Geometry: see drawing. Coordinates: mm, zero at the bounding-box minimum. Round coordinates to 2 decimals unless told otherwise and drop trailing zeros. Write each loop counter-clockwise with the first axis right and the second up, starting at its lowest first coordinate (ties: lowest second). Pieces come first, ordered by that corner, then holes. Notation, with made-up numbers: (45, 42.5) -> (94, 42.5) arc R8 cw to (94, 49.5) -> close; hole circle Ø1 at (-4, 57.25). An arc over 180 degrees is marked (long way). Write item = value, one per line.
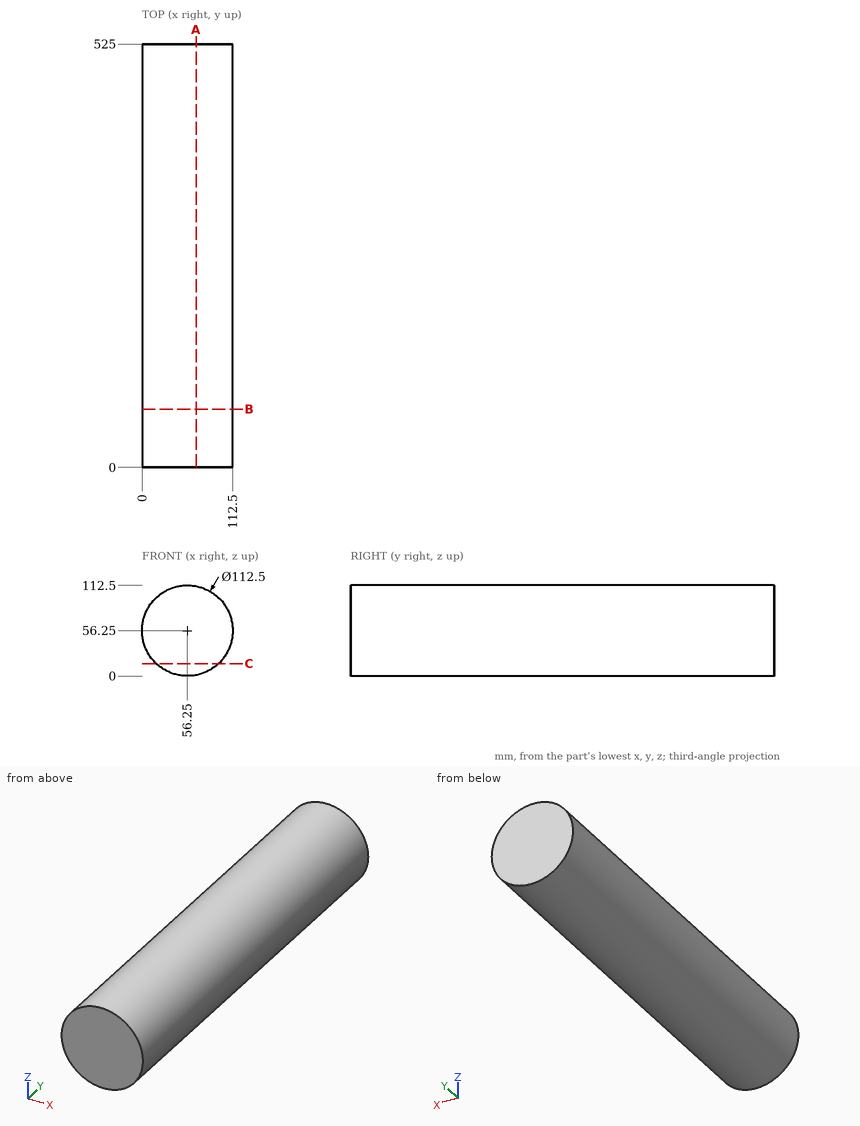
1) Cut plane C-C (z = 15.5). Return the cut outline in (x, y) (3 decimals).
Solutions:
outline = (17.475, 0) -> (95.025, 0) -> (95.025, 525) -> (17.475, 525) -> close
2) Line query: L1, parallel to X at y = 195, z = 103.5; L2, parallel to X at y = 356.5, z = 20; L3, parallel to Z at x = 83, y = 257.5. Output: solid intervals per line, ascending. Write a range as from..to.
Solutions:
L1 = 25.73..86.77
L2 = 13.24..99.26
L3 = 6.77..105.73
3) Cut plane A-A (x = 67). Return the cut outline in (y, z).
Solutions:
outline = (0, 1.04) -> (525, 1.04) -> (525, 111.46) -> (0, 111.46) -> close
4) First-contact query: P1, Ø4, axis at y = 106, z = 100, coming from the +X side; P2, Ø2, axis at x = 16.5, y = 417, coming from the +Z side; P3, Ø5, axis at x = 77, y = 368, coming from the -Z side. Flat tips, straight axial feed; report the tip coordinate or a pass-through.
Solutions:
P1 = 93.95
P2 = 97.02
P3 = 3.04
5) Cut plane B-B (y = 72). Return the cut outline in (x, z), and give its area (3 significant figures).
Solutions:
outline = circle Ø112.5 at (56.25, 56.25)
area = 9,940 mm^2
